Here's how the part is built. I have some questions about the finished solid (model axes, mm). Coordinates: 2 decimals unless noted, no trailing zeros. Order: outer loops, then holes, each group sorted by start corner. A loop starts at its lowest first (then second) coordinate and runs counter-clockwise, first axis right, second up. Notation, with made-up numbers: M 40,5.5 L 65,5.5 A26 ccw 65,23.5 Z; hole C 62.5,11 d8. An arc over 180 degrees is marked long. One line per question, with ' | ' between items. Start each with the question number.
Autodesk Inventor part; units mm, degrees
ref_plane "YZ Plane" through (0, 0, 0) normal (1, 0, 0) x (0, 1, 0)
ref_plane "XZ Plane" through (0, 0, 0) normal (0, 1, 0) x (-1, 0, 0)
ref_plane "XY Plane" through (0, 0, 0) normal (0, 0, 1) x (1, 0, 0)
sketch "Szkic1" plane through (0, 0, 0) normal (0, 1, 0) x (-1, 0, 0)
  line L0 (0, 0) -> (0, -5)
  line L1 (0, -5) -> (-6, -5)
  line L2 (-6, -5) -> (-6, -3.5)
  line L3 (-6, -3.5) -> (-1.5, -3.5)
  line L4 (-1.5, -3.5) -> (-1.5, 0)
  line L5 (0, 0) -> (-1.5, 0)
  line L6 (0, 0) -> (0, 5)
  line L7 (0, 5) -> (-6, 5)
  line L8 (-6, 5) -> (-6, 3.5)
  line L9 (-6, 3.5) -> (-1.5, 3.5)
  line L10 (-1.5, 3.5) -> (-1.5, 0)
  dimension "d0" = 5
  dimension "d1" = 6
  dimension "d3" = 1.5
  dimension "d41" = 1.5
extrude "Wyciągnięcie proste1" add sketch "Szkic1" along normal blind 1000
sketch "Szkic2" plane through (1.5, 0, -3.5) normal (1, 0, 0) x (0, 0, -1)
  line L0 (-3.5, 0) -> (-3.5, 1000)
  line L1 (-7, 0) -> (-7, 1000)
  line L2 (-3.5, 1000) -> (-3.5, 995)
  line L3 (-3.5, 995) -> (-3.5, 795)
  line L4 (-3.5, 795) -> (-3.5, 795)
  line L5 (-3.5, 795) -> (-3.5, 695)
  line L6 (-3.5, 695) -> (-3.5, 595)
  line L7 (-3.5, 595) -> (-3.5, 495)
  line L8 (-7, 0) -> (0, 0)
  line L9 (-3.5, 595) -> (-3.5, 395)
  line L10 (-3.5, 395) -> (-3.5, 195)
  line L11 (-3.5, 195) -> (-3.5, 0)
  line L12 (-3.5, 0) -> (-3.5, 5)
  dimension "d7" = 5
  dimension "d13" = 200
  dimension "d14" = 200
  dimension "d16" = 200
  dimension "d17" = 200
  dimension "d18" = 195
  dimension "d19" = 5
sketch "Szkic3" plane through (6, 0, 5) normal (0, 0, 1) x (1, 0, 0)
  line L0 (0, 0) -> (-6, 0)
  line L1 (-3, 0) -> (-3, 5)
  line L2 (-3, 5) -> (-3, 205)
  line L3 (-3, 205) -> (-3, 405)
  line L4 (-3, 405) -> (-3, 605)
  line L5 (-3, 605) -> (-3, 805)
  line L6 (-3, 805) -> (-3, 1000)
  line L7 (-3, 1000) -> (-3, 995)
  dimension "d27" = 5
  dimension "d28" = 200
  dimension "d29" = 200
  dimension "d30" = 200
  dimension "d31" = 200
  dimension "d32" = 195
  dimension "d33" = 5
hole "Otwór2" at (3, 5, 5) at (3, 205, 5) at (3, 405, 5) at (3, 605, 5) at (3, 805, 5) at (3, 995, 5) direction (0, 0, -1) diameter 2.5 end through all countersink diameter 3 countersink angle 90
properties part number "prowadnica_profil_c_CPY"
1. I need wall thicknesses on line 1 (Z direction, x = 4.8, y = 815); line 2 (X direction, y = 205, z = -4.6); line 3 (X direction, y = 312, z = 0.75). Which ranges of each line are inside material? Lowest first, please.
2. Imagine slicing it at C-C (z = 1.75). List the corners of the cut face in (x, y) for me.
3. Imagine slicing it at B-B (x = 3). Count the separate pieces of the cut face and the enclosed holes in it, then the cut area to 3 significant figures.
4. Imagine slicing it at A-A (y = 245). List the corners of the cut face in (x, z) for me.
5. Will these pins go through, and if not, where does the flat tip stop? pin 1 (2 mm diameter, centred on y = 605, z = 0.5, fed in from +X); pin 2 (3 mm diameter, centred on x = 3, y = 5, fed in from -Z).
Entries:
1) line 1: -5 to -3.5, 3.5 to 5 | line 2: 0 to 1.75, 4.25 to 6 | line 3: 0 to 1.5
2) outline: M 0,0 L 1.5,0 L 1.5,1000 L 0,1000 Z
3) separate pieces: 14 | enclosed holes: 0 | area: 2,950 mm²
4) outline: M 0,-5 L 6,-5 L 6,-3.5 L 1.5,-3.5 L 1.5,3.5 L 6,3.5 L 6,5 L 0,5 Z
5) pin 1: x = 1.5 | pin 2: z = -5
